```python
from build123d import *

# Parameters (mm, degrees)
SKETCH1_W           = 350
SKETCH1_H           = 350
BOSS_EXTRUDE1_DEPTH = 30
SKETCH2_R           = 105.873487711
BOSS_EXTRUDE2_DEPTH = 12
CUT_EXTRUDE1_DEPTH  = 12
CUT_EXTRUDE3_DEPTH  = 394.559398312


with BuildPart() as part:
    # Sketch1 → Boss-Extrude1 (new body)
    with BuildSketch(Plane.XY):
        Rectangle(SKETCH1_W, SKETCH1_H)
    extrude(amount=BOSS_EXTRUDE1_DEPTH)

    # Sketch2 → Boss-Extrude2 (add)
    with BuildSketch(Plane.XY.offset(30)):
        Circle(SKETCH2_R)
    extrude(amount=BOSS_EXTRUDE2_DEPTH)

    # Sketch3 → Cut-Extrude1 (cut)
    with BuildSketch(Plane.XY.offset(42)):
        with BuildLine():
            Line((-4.5, 18.356470249), (-4.5, 33.356470249))
            Line((-4.5, 33.356470249), (4.5, 33.356470249))
            Line((4.5, 33.356470249), (4.5, 18.356470249))
            ThreePointArc((4.5, 18.356470249), (18.9, 0), (4.5, -18.356470249))
            Line((4.5, -18.356470249), (4.5, -33.356470249))
            Line((4.5, -33.356470249), (-4.5, -33.356470249))
            Line((-4.5, -33.356470249), (-4.5, -18.356470249))
            ThreePointArc((-4.5, -18.356470249), (-18.9, 0), (-4.5, 18.356470249))
        make_face()
    extrude(amount=-CUT_EXTRUDE1_DEPTH, mode=Mode.SUBTRACT)

    # Sketch5 → Cut-Extrude3 (cut, through all)
    with BuildSketch(Plane(origin=(0, 175, 0), x_dir=(1, 0, 0), z_dir=(0, 1, 0))):
        Polygon((-145, 0), (-155, 0), (-155, -10), (-160, -10), (-160, -25), (-140, -25), (-140, -10), (-145, -10), align=None)
        Polygon((-95, 0), (-105, 0), (-105, -10), (-110, -10), (-110, -25), (-90, -25), (-90, -10), (-95, -10), align=None)
        Polygon((-45, 0), (-55, 0), (-55, -10), (-60, -10), (-60, -25), (-40, -25), (-40, -10), (-45, -10), align=None)
        Polygon((5, 0), (-5, 0), (-5, -10), (-10, -10), (-10, -25), (10, -25), (10, -10), (5, -10), align=None)
        Polygon((55, 0), (45, 0), (45, -10), (40, -10), (40, -25), (60, -25), (60, -10), (55, -10), align=None)
        Polygon((105, 0), (95, 0), (95, -10), (90, -10), (90, -25), (110, -25), (110, -10), (105, -10), align=None)
        Polygon((155, 0), (145, 0), (145, -10), (140, -10), (140, -25), (160, -25), (160, -10), (155, -10), align=None)
    extrude(amount=-CUT_EXTRUDE3_DEPTH, mode=Mode.SUBTRACT)


solid = part.part
```
Geometry check sheet. Reference: the model listing, model coordinates, mm. A direction names the side the tool comes from. Round coordinates to 2 decimals unless told otherwise and drop trailing zeros. Order: outer loops, then holes, each group sorted by start corner. A loop starts at its lowest first (then second) coordinate and runs counter-clockwise, first axis right, second up. Notation, with made-up numbers: (-4.5, 66) - (13.5, 66) arc R19 ccw to (13.5, 91) - close; hole circle Ø4 at (64.25, 47.5). An arc over 180 degrees is marked (long way). Use a Markdown table: item, result. Add a question column.
1) Set-up check for faces 1 (the flat face through (-75, 2, 0)), 2 (the flat face through (-145, 2, 5)), 3 (the flat face through (0, 2, 25)): record each of +Z, -Z, +X, -X, +Y, -Y from which the full face is reachable in a straight line by a thin tool's end or side.
2) Section check A-A (z = 34.5). Record the cut outline in (x, y), then the cut area to 3 significant figures.
3) Thickness scan on line 1 along Z through (x, y) = (-107, -28.5); line 2 along Z through (x, y) = (128.5, -24.5); line 3 along X through (y, z) = (26.5, 40). Record the ranges inside material, lowest first.
4) Gauge pin test, flat ends, axial feed: P1, Ø5.5, axis at x = -142.5, y = 86, coming from the +Z side; P2, Ø5, axis at y = 9, z = 35.5, coming from the +X side; P3, Ø16, axis at x = 46, y = -57, coming from the -Z side; P4, Ø5, axis at y = 26.5, z = 36, coming from the -X side. Record the tip position at first contact, or that the pin passes through.
5) Section check B-B (z = 6). Count the separate pieces of the cut face and the enclosed holes in it, then the cut area to 3 significant figures.
6) Section check D-D (x = -85). Record the cut outline in (y, z).
7) Section check C-C (x = 0). Record the cut outline in (y, z).
8) Mould release check, pull along Z, two halves, no side actions. Record for faces 4 (the flat face through (10, 2, 18)), 5 (the flat face through (-55, 2, 5)), 6 (the flat face through (165, 2, 0)): released by +Z, released by -Z, zero draft, split by the parting line, or undercut.
Established:
| question | item | result |
|---|---|---|
| 1 | face 1 | -Z, +X, -X, +Y, -Y |
| 1 | face 2 | -Z, +Y, -Y |
| 1 | face 3 | +Y, -Y |
| 2 | outline | circle Ø211.75 at (0, 0); hole (-4.5, -33.36) - (4.5, -33.36) - (4.5, -18.36) arc R18.9 ccw to (4.5, 18.36) - (4.5, 33.36) - (-4.5, 33.36) - (-4.5, 18.36) arc R18.9 ccw to (-4.5, -18.36) - close |
| 2 | area | 33,800 mm2 |
| 3 | line 1 | 0 to 10, 25 to 30 |
| 3 | line 2 | 0 to 30 |
| 3 | line 3 | -102.5 to -4.5, 4.5 to 102.5 |
| 4 | P1 | z = 30 |
| 4 | P2 | x = 105.67 |
| 4 | P3 | z = 0 |
| 4 | P4 | x = -103.12 |
| 5 | separate pieces | 8 |
| 5 | enclosed holes | 0 |
| 5 | area | 98,000 mm2 |
| 6 | outline | (-175, 0) - (175, 0) - (175, 30) - (63.12, 30) - (63.12, 42) - (-63.12, 42) - (-63.12, 30) - (-175, 30) - close |
| 7 | outline | (-175, 25) - (175, 25) - (175, 30) - (105.87, 30) - (105.87, 42) - (33.36, 42) - (33.36, 30) - (-33.36, 30) - (-33.36, 42) - (-105.87, 42) - (-105.87, 30) - (-175, 30) - close |
| 8 | face 4 | undercut |
| 8 | face 5 | zero draft |
| 8 | face 6 | released by -Z |
